```python
from build123d import *

# Parameters (mm, degrees)
BOSS_EXTRUDE1_DEPTH = 6.35


with BuildPart() as part:
    # Sketch1 → Boss-Extrude1 (new body)
    with BuildSketch(Plane.XY):
        with BuildLine():
            ThreePointArc((19.09558361, -27.286492755), (15.377016657, -28.688589019), (12.38097626, -31.299595732))
            ThreePointArc((12.38097626, -31.299595732), (11.754813891, -32.585358585), (11.743487691, -34.015441499))
            ThreePointArc((11.743487691, -34.015441499), (14.816954296, -41.959391499), (20.1598835, -48.593066656))
            ThreePointArc((20.1598835, -48.593066656), (21.404034733, -49.298299337), (22.830619211, -49.398908245))
            ThreePointArc((22.830619211, -49.398908245), (26.589837552, -48.109764507), (29.663372012, -45.590439192))
            ThreePointArc((29.663372012, -45.590439192), (32.39282557, -43.727845578), (35.689842925, -43.506829177))
            ThreePointArc((35.689842925, -43.506829177), (38.793733625, -43.816700713), (41.897624325, -43.506829177))
            ThreePointArc((41.897624325, -43.506829177), (45.194641681, -43.727845578), (47.924095238, -45.590439192))
            ThreePointArc((47.924095238, -45.590439192), (50.997629698, -48.109764507), (54.75684804, -49.398908245))
            ThreePointArc((54.75684804, -49.398908245), (56.183432518, -49.298299337), (57.427583751, -48.593066656))
            ThreePointArc((57.427583751, -48.593066656), (62.770512955, -41.959391499), (65.84397956, -34.015441499))
            ThreePointArc((65.84397956, -34.015441499), (65.83265336, -32.585358585), (65.206490991, -31.299595732))
            ThreePointArc((65.206490991, -31.299595732), (62.210450594, -28.688589019), (58.491883641, -27.286492755))
            ThreePointArc((58.491883641, -27.286492755), (55.514103476, -25.854013443), (53.67418898, -23.109220856))
            ThreePointArc((53.67418898, -23.109220856), (52.390600252, -20.266236892), (50.57029828, -17.733124463))
            ThreePointArc((50.57029828, -17.733124463), (49.11319542, -14.767315476), (49.361522028, -11.47224255))
            ThreePointArc((49.361522028, -11.47224255), (50.006554521, -7.550820971), (49.243376577, -3.650670519))
            ThreePointArc((49.243376577, -3.650670519), (48.442954467, -2.465516575), (47.210129434, -1.740666341))
            ThreePointArc((47.210129434, -1.740666341), (38.793733625, -0.430391499), (30.377337817, -1.740666341))
            ThreePointArc((30.377337817, -1.740666341), (29.144512783, -2.465516575), (28.344090674, -3.650670519))
            ThreePointArc((28.344090674, -3.650670519), (27.58091273, -7.550820971), (28.225945223, -11.47224255))
            ThreePointArc((28.225945223, -11.47224255), (28.47427183, -14.767315476), (27.01716897, -17.733124463))
            ThreePointArc((27.01716897, -17.733124463), (25.196866999, -20.266236892), (23.91327827, -23.109220856))
            ThreePointArc((23.91327827, -23.109220856), (22.073363775, -25.854013443), (19.09558361, -27.286492755))
        make_face()
    extrude(amount=BOSS_EXTRUDE1_DEPTH)


solid = part.part
```
For this review, take the finished solid that the model builds, in its own axes (mm). A direction names the side the tool comes from. Round coordinates to 2 decimals unless told otherwise and drop trailing zeros. Loops run counter-clockwise (first coordinate to the right, second up) from the corner with the lowest first, then second, coordinate; pieces in that order, holes last.
Q1. Add section C-C on x = 16.5. Write out the cut boundary in (y, z), plus the area to 3 significant figures.
Result sheet:
outline: (-44.53, 0) - (-28.1, 0) - (-28.1, 6.35) - (-44.53, 6.35) - close
area: 104 mm2
Q2. To check wall thickness, follow line 1 along X through (y, z) = (-45.5, 2); line 2 along Y through (x, z) = (14, 2); line 3 along Y through (x, z) = (36.5, 4.25). State the ranges of each line that lie inside material, in increasing order.
Result sheet:
line 1: x = 17.25 to 29.74, 47.85 to 60.34
line 2: y = -40.44 to -29.66
line 3: y = -43.65 to -0.53
Q3. Insertion check: pin 1 Ø2 at (x, z) = (20, 2) entering from -Y; pin 2 Ø1 at (x, z) = (58.5, 3) entering from -Y; pin 3 Ø1.5 at (y, z) = (-43, 4) entering from +X. Each pin has a flat end and moves straight along its axis. Give the tip position at first contact, or say it passes through.
Result sheet:
pin 1: stops at y = -49.15
pin 2: stops at y = -48.06
pin 3: stops at x = 62.6
Q4. Mouldability with a two-part tool opening along Y and no side actions: class faces 3 (the face through (11.76, -32.57, 3.13)), 4 (the face through (25.22, -20.23, 3.13)), 5 (the face through (27.58, -7.49, 3.13)), 6 (the face through (50.949, -48.082, 3.131)) as +Y half, -Y half, draft (parallel to the pull), parting line (faces both ways), or undercut.
Result sheet:
face 3: parting line
face 4: +Y half
face 5: undercut
face 6: -Y half
Q5. Add section A-A on y = -45. Write out the cut boundary in (x, z).
Result sheet:
outline: (16.85, 0) - (30.24, 0) - (30.24, 6.35) - (16.85, 6.35) - close; (47.35, 0) - (60.74, 0) - (60.74, 6.35) - (47.35, 6.35) - close
Q6. Add section B-B on z = 3.75. Write out the cut boundary in (x, y), plus the area to 3 significant figures.
Result sheet:
outline: (11.74, -34.02) arc R27.69 ccw to (20.16, -48.59) arc R3.24 ccw to (22.83, -49.4) arc R11.21 ccw to (29.66, -45.59) arc R6.29 cw to (35.69, -43.51) arc R15.7 ccw to (41.9, -43.51) arc R6.29 cw to (47.92, -45.59) arc R11.21 ccw to (54.76, -49.4) arc R3.24 ccw to (57.43, -48.59) arc R27.69 ccw to (65.84, -34.02) arc R3.24 ccw to (65.21, -31.3) arc R11.21 ccw to (58.49, -27.29) arc R6.29 cw to (53.67, -23.11) arc R15.7 ccw to (50.57, -17.73) arc R6.29 cw to (49.36, -11.47) arc R11.21 ccw to (49.24, -3.65) arc R3.24 ccw to (47.21, -1.74) arc R27.69 ccw to (30.38, -1.74) arc R3.24 ccw to (28.34, -3.65) arc R11.21 ccw to (28.23, -11.47) arc R6.29 cw to (27.02, -17.73) arc R15.7 ccw to (23.91, -23.11) arc R6.29 cw to (19.1, -27.29) arc R11.21 ccw to (12.38, -31.3) arc R3.24 ccw to start
area: 1,580 mm2
Q7. Machinability: for faces 1 (the face through (26.541, -48.137, 3.131)), 2 (the face through (28.483, -14.721, 3.131)), which of the approach directions +Z, -Z, +X, -X, +Y, -Y give a long, thin tool a straight path to every point of the face, cutting with its end or side? Answer none if there is none.
Result sheet:
face 1: +Z, -Z, -Y
face 2: +Z, -Z, -X
Q8. Add section D-D on y = -13. Write out the cut boundary in (x, z).
Result sheet:
outline: (28.56, 0) - (49.03, 0) - (49.03, 6.35) - (28.56, 6.35) - close
